Verification items for the finished model (mm, model axes). Face numbers are marked on the shaded views. A direction names the side the tool comes from. Coordinates: 2 decimals unless noted, no trailing zeros. Write each loop counter-clockwise with the first axis right and the second up, starting at its lowest first coordinate (ties: lowest second). Pieces come first, ordered by that corner, then holes. Notation, with made-up numbers: (58.5, -25) -> (102.5, -25) arc R27 ccw to (102.5, -1) -> close; hole circle Ø4 at (71.25, 39.25). An arc over 180 degrees is marked (long way). Answer in a Markdown table with one row per item.
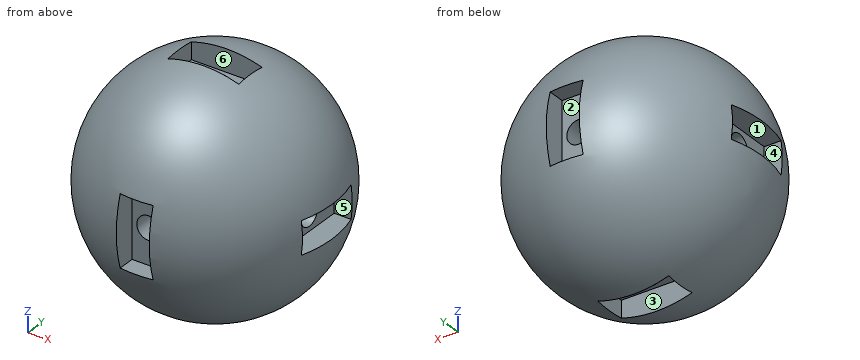
```python
from build123d import *

# Parameters (mm, degrees)
F3_W      = 7
F3_H      = 15
F4_DEPTH  = 5
F5_R      = 2.5
F6_DEPTH  = 45.001
F8_W      = 15
F8_H      = 7
F9_DEPTH  = 5
F10_R     = 2.5
F11_DEPTH = 44.754787589
F13_W     = 15
F13_H     = 7
F14_DEPTH = 5
F15_R     = 2.5
F16_DEPTH = 44.754787589


# Not quite as in the source:
# - a pattern or mirror of a feature is missing from the dataset's text; its kind, count and spacing are read off the source's solid


with BuildPart() as f1:
    # F0 (on Front) → F1 (revolve)
    with BuildSketch(Plane.XZ):
        with BuildLine():
            Line((0, -25), (0, 25))
            ThreePointArc((0, 25), (-25, 0), (0, -25))
        make_face()
    revolve(axis=Axis((0, 0, 0), (0, 0, -1)))

    # F3 (on offset) → F4 (cut)
    with BuildSketch(Plane.XZ.offset(25)):
        Rectangle(F3_W, F3_H)
    f4 = extrude(amount=-F4_DEPTH, mode=Mode.SUBTRACT)

    # F4_copies: F4 across plane
    add(f4.mirror(Plane.ZX), mode=Mode.SUBTRACT)

    # F5 (on face) → F6 (cut, through all)
    with BuildSketch(Plane.XZ.offset(20)):
        Circle(F5_R)
    extrude(amount=-F6_DEPTH, mode=Mode.SUBTRACT)

    # F8 (on offset) → F9 (cut)
    with BuildSketch(Plane.XY.offset(25)):
        Rectangle(F8_W, F8_H)
    f9 = extrude(amount=-F9_DEPTH, mode=Mode.SUBTRACT)

    # F9_copies: F9 across plane
    add(f9.mirror(Plane(origin=(0, 0, 0), x_dir=(-1, 0, 0), z_dir=(0, 0, -1))), mode=Mode.SUBTRACT)

    # F10 (on face) → F11 (cut, through all)
    with BuildSketch(Plane.XY.offset(20)):
        Circle(F10_R)
    extrude(amount=-F11_DEPTH, mode=Mode.SUBTRACT)

    # F13 (on offset) → F14 (cut)
    with BuildSketch(Plane.YZ.offset(25)):
        Rectangle(F13_W, F13_H)
    f14 = extrude(amount=-F14_DEPTH, mode=Mode.SUBTRACT)

    # F14_copies: F14 across plane
    add(f14.mirror(Plane(origin=(0, 0, 0), x_dir=(0, 0, -1), z_dir=(-1, 0, 0))), mode=Mode.SUBTRACT)

    # F15 (on face) → F16 (cut, through all)
    with BuildSketch(Plane.YZ.offset(20)):
        Circle(F15_R)
    extrude(amount=-F16_DEPTH, mode=Mode.SUBTRACT)


solid = f1.part
```
1. Section check B-B, the plane x = 0. Record the boundary of the cut face in (y, z), plus the area to 3 significant figures.
Geometry says:
| item | result |
|---|---|
| outline | (-23.85, -7.5) arc R25 ccw to (-3.5, -24.75) -> (-3.5, -20) -> (-2.5, -20) -> (-2.5, -2.5) -> (-20, -2.5) -> (-20, -7.5) -> close; (-23.85, 7.5) -> (-20, 7.5) -> (-20, 2.5) -> (-2.5, 2.5) -> (-2.5, 20) -> (-3.5, 20) -> (-3.5, 24.75) arc R25 ccw to start; (2.5, -20) -> (3.5, -20) -> (3.5, -24.75) arc R25 ccw to (23.85, -7.5) -> (20, -7.5) -> (20, -2.5) -> (2.5, -2.5) -> close; (2.5, 2.5) -> (20, 2.5) -> (20, 7.5) -> (23.85, 7.5) arc R25 ccw to (3.5, 24.75) -> (3.5, 20) -> (2.5, 20) -> close |
| area | 1,380 mm^2 |
2. Depth check by flat-ended pin: P1, Ø1.9, axis at x = 0.5, y = -21.5, coming from the -Z side; P2, Ø10, axis at x = 14.5, z = 18, coming from the +Y side; P3, Ø1.9, axis at x = 0, y = -21, coming from the +Z side. Enter the tip coordinate at first touch or a pass-through.
Geometry says:
| item | result |
|---|---|
| P1 | z = -14.23 |
| P2 | y = 17.23 |
| P3 | z = 14.93 |
3. Section check A-A, the plane y = 0. Record the boundary of the cut face in (x, z), plus the area to 3 significant figures.
Geometry says:
| item | result |
|---|---|
| outline | (-24.75, -3.5) arc R25 ccw to (-7.5, -23.85) -> (-7.5, -20) -> (-2.5, -20) -> (-2.5, -2.5) -> (-20, -2.5) -> (-20, -3.5) -> close; (-24.75, 3.5) -> (-20, 3.5) -> (-20, 2.5) -> (-2.5, 2.5) -> (-2.5, 20) -> (-7.5, 20) -> (-7.5, 23.85) arc R25 ccw to start; (2.5, -20) -> (7.5, -20) -> (7.5, -23.85) arc R25 ccw to (24.75, -3.5) -> (20, -3.5) -> (20, -2.5) -> (2.5, -2.5) -> close; (2.5, 2.5) -> (20, 2.5) -> (20, 3.5) -> (24.75, 3.5) arc R25 ccw to (7.5, 23.85) -> (7.5, 20) -> (2.5, 20) -> close |
| area | 1,380 mm^2 |
4. Section check D-D, the plane z = 15.5. Record the boundary of the cut face in (x, y), plus the area to 3 significant figures.
Geometry says:
| item | result |
|---|---|
| outline | circle Ø39.23 at (0, 0); hole circle Ø5 at (0, 0) |
| area | 1,190 mm^2 |
5. Mould release check, pull along X, two halves, no side actions. Record for the marked faces 1 and 2: released by +X, released by -X, zero draft, split by the parting line, or undercut.
Geometry says:
| item | result |
|---|---|
| face 1 | zero draft |
| face 2 | undercut |
6. Thickness scan on line 1 (Z direction, x = 6, y = 0); line 2 (Z direction, x = 0, y = 6); line 3 (X direction, y = 0, z = -7). Record the ranges inside material, lowest first. Write a range as from..to.
Geometry says:
| item | result |
|---|---|
| line 1 | -20..-2.5, 2.5..20 |
| line 2 | -24.27..-2.5, 2.5..24.27 |
| line 3 | -24..-2.5, 2.5..24 |
7. Tool access check on the marked faces 3, 4, 5 and 6. Record the directions out of +Z, -Z, +X, -X, +Y, -Y that give a thin tool (end or side, any length) a straight path to the whole face; none if there is none.
Geometry says:
| item | result |
|---|---|
| face 3 | -Z |
| face 4 | -X |
| face 5 | +X |
| face 6 | +Z |
8. Section check C-C, the plane y = -6.5. Record the boundary of the cut face in (x, z), plus the area to 3 significant figures.
Geometry says:
| item | result |
|---|---|
| outline | (-23.89, -3.5) arc R24.14 ccw to (23.89, -3.5) -> (20, -3.5) -> (20, 3.5) -> (23.89, 3.5) arc R24.14 ccw to (-23.89, 3.5) -> (-20, 3.5) -> (-20, -3.5) -> close; hole circle Ø5 at (0, 0) |
| area | 1,750 mm^2 |
